Part model, mm, in its own coordinate system. A direction names the side the tool comes from. Round coordinates to 2 decimals unless told otherwise and drop trailing zeros. Write each loop counter-clockwise with the first axis right and the second up, starting at its lowest first coordinate (ties: lowest second). Pieces come first, ordered by that corner, then holes. Notation, with made-up numbers: (33, 86.5) -> (58, 86.5) arc R14 ccw to (58, 111.5) -> close; hole circle Ø1 at (26, 67.5). An arc over 180 degrees is marked (long way). Return JSON: item names as keys, results as strings. Group by question number.
(1) Mould opens along X. For faces 5 (the flat face through (-7.307, 0, -6)), 6 (the flat face through (0, 0, 5.1)), 7 (the flat face through (0, -3.2, 0)), 8 (the flat face through (8.2, 0, 7)) say: +X half, -X half, draft (parallel to the pull), parting line (faces both ways), or undercut.
(2) Saw through at A-A (x = -4.8). List the corners of the cut face in (y, z), plus the area to 3 significant figures.
(3) Drill centre lines: L1, parallel to X at y = -2, z = 2.6 (3 decimals); L2, parallel to X at y = 1.5, z = 7.75; L3, parallel to Z at x = 4.7, y = 0 (3 decimals). Where is each one in solid material? Low to high. Write a range as from..to.
(4) Drop flat-ended pins along their axis: pin 1 Ø2.5 at (y, z) = (0, 7.5) entering from -X; pin 2 Ø1.6 at (y, z) = (0, 7.5) entering from +X; pin 3 Ø1.1 at (x, y) = (-2.5, 0.5) entering from +Z. Give the stop position or say it passes through.
(5) Saw through at B-B (z = 6). List the corners of the cut face in (x, y).
(6) Saw through at D-D (x = -1). List the corners of the cut face in (y, z).
(7) Tool access for faces 1 (the cylindrical face through (-3.296, 0.024, -5.607)), 2 (the flat face through (1, 1.8, -6)), 3 (the flat face through (0.5, 0, 7)), 4 (the flat face through (1, -1.8, -6)): list every direction of +Z, -Z, +X, -X, +Y, -Y with a clear straight run to the whole face (end or side of a thin tool).
(8) Saw through at C-C (y = 2.5). List the corners of the cut face in (x, z) (3 decimals).
from build123d import *

# Parameters (mm, degrees)
SKETCH1_W               = 19.8
SKETCH1_H               = 10.2
BOSS_EXTRUDE1_DEPTH     = 3.2
SKETCH2_R               = 1.25
SKETCH2_R_2             = 1.175
CUT_EXTRUDE1_DEPTH      = 4.2
CUT_EXTRUDE1_DEPTH_BACK = 4.2
BOSS_EXTRUDE2_DEPTH     = 1.8
SKETCH4_W               = 0.4
SKETCH4_H               = 3.2
BOSS_EXTRUDE3_DEPTH     = 3.9
LPATTERN1_COUNT         = 2
LPATTERN1_PITCH         = 8.8
LPATTERN2_COUNT         = 2
LPATTERN2_PITCH         = 16.1
SKETCH5_R               = 0.507136528
BOSS_EXTRUDE4_DEPTH     = 1.7


with BuildPart() as part:
    # Sketch1 → Boss-Extrude1 (new body, symmetric)
    with BuildSketch(Plane(origin=(0, 0, 0), x_dir=(1, 0, 0), z_dir=(0, 1, 0))):
        Rectangle(SKETCH1_W, SKETCH1_H)
    extrude(amount=BOSS_EXTRUDE1_DEPTH, both=True)

    # Sketch2 → Cut-Extrude1 (cut, two sides)
    with BuildSketch(Plane(origin=(0, 0, 0), x_dir=(1, 0, 0), z_dir=(0, 1, 0))) as cut_extrude1_sk:
        with Locations((-4.8, -2.6)):
            Circle(SKETCH2_R)
        with Locations((4.7, -2.6)):
            Circle(SKETCH2_R_2)
    extrude(amount=CUT_EXTRUDE1_DEPTH, mode=Mode.SUBTRACT)
    extrude(cut_extrude1_sk.sketch, amount=-CUT_EXTRUDE1_DEPTH_BACK, mode=Mode.SUBTRACT)

    # Sketch3 → Boss-Extrude2 (add, symmetric)
    with BuildSketch(Plane(origin=(0, 0, 0), x_dir=(1, 0, 0), z_dir=(0, 1, 0))):
        Polygon((-7.306635191, 5.1), (-7.306635191, 6.2), (9.7, 6.2), (9.7, 5.775620591), (-6.694229351, 5.775620591), (-6.694229351, 5.1), align=None)
    extrude(amount=BOSS_EXTRUDE2_DEPTH, both=True)

    # Sketch4 → Boss-Extrude3 (add)
    with BuildSketch(Plane.XY.offset(5.1)):
        with Locations((-8.1, 0)):
            Rectangle(SKETCH4_W, SKETCH4_H)
    boss_extrude3 = extrude(amount=BOSS_EXTRUDE3_DEPTH)

    # LPattern1: Boss-Extrude3 ×2
    with Locations(*[(i * LPATTERN1_PITCH, 0, 0) for i in range(1, LPATTERN1_COUNT)]):
        add(boss_extrude3)

    # LPattern2: Boss-Extrude3 ×2
    with Locations(*[(i * LPATTERN2_PITCH, 0, 0) for i in range(1, LPATTERN2_COUNT)]):
        add(boss_extrude3)

    # Sketch5 → Boss-Extrude4 (add, symmetric)
    with BuildSketch(Plane(origin=(0, 0, 0), x_dir=(1, 0, 0), z_dir=(0, 1, 0))):
        with Locations((-3.307427246, 5.1)):
            Circle(SKETCH5_R)
    extrude(amount=BOSS_EXTRUDE4_DEPTH, both=True)


solid = part.part
Computed values:
{
 "1": {"face 5": "-X half", "face 6": "undercut", "face 7": "draft", "face 8": "+X half"},
 "2": {"outline": "(-3.2, -5.1) -> (3.2, -5.1) -> (3.2, 1.35) -> (-3.2, 1.35) -> close; (-3.2, 3.85) -> (3.2, 3.85) -> (3.2, 5.1) -> (-3.2, 5.1) -> close; (-1.8, -6.2) -> (1.8, -6.2) -> (1.8, -5.78) -> (-1.8, -5.78) -> close", "area": "50.8 mm2"},
 "3": {"L1": "-9.9..-6.05, -3.55..3.525, 5.875..9.9", "L2": "-8.3..-7.9, 0.5..0.9, 7.8..8.2", "L3": "-6.2..-5.776, -5.1..1.425, 3.775..5.1"},
 "4": {"pin 1": "x = -8.3", "pin 2": "x = 8.2", "pin 3": "z = 5.1"},
 "5": {"outline": "(-8.3, -1.6) -> (-7.9, -1.6) -> (-7.9, 1.6) -> (-8.3, 1.6) -> close; (0.5, -1.6) -> (0.9, -1.6) -> (0.9, 1.6) -> (0.5, 1.6) -> close; (7.8, -1.6) -> (8.2, -1.6) -> (8.2, 1.6) -> (7.8, 1.6) -> close"},
 "6": {"outline": "(-3.2, -5.1) -> (3.2, -5.1) -> (3.2, 5.1) -> (-3.2, 5.1) -> close; (-1.8, -6.2) -> (1.8, -6.2) -> (1.8, -5.78) -> (-1.8, -5.78) -> close"},
 "7": {"face 1": "+Y, -Y", "face 2": "-Z, +X, -X, +Y", "face 3": "+Z, +Y, -Y", "face 4": "-Z, +X, -X, -Y"},
 "8": {"outline": "(-9.9, -5.1) -> (9.9, -5.1) -> (9.9, 5.1) -> (-9.9, 5.1) -> close; hole circle Ø2.5 at (-4.8, 2.6); hole circle Ø2.35 at (4.7, 2.6)"}
}
